```python
from build123d import *

# Parameters (mm, degrees)
CROQUIS1_W                 = 105
CROQUIS1_H                 = 30
CROQUIS1_R                 = 5
SALIENTE_EXTRUIR1_DEPTH    = 70
CORTAR_EXTRUIR1_DEPTH      = 30
CORTAR_EXTRUIR1_DEPTH_BACK = 30
CROQUIS2_R                 = 40
CROQUIS3_R                 = 5
CORTAR_EXTRUIR2_DEPTH      = 30
CROQUIS4_W                 = 55
CROQUIS4_H                 = 60
CORTAR_EXTRUIR3_DEPTH      = 30


with BuildPart() as part:
    # Croquis1 → Saliente-Extruir1 (new body)
    with BuildSketch(Plane(origin=(0, 0, 0), x_dir=(1, 0, 0), z_dir=(0, 1, 0))):
        with Locations((14.264686972, 6.108870968)):
            Rectangle(CROQUIS1_W, CROQUIS1_H)
        with Locations(Location((56.764686972, 6.108870968, 0), (0, 0, 270))):
            Circle(CROQUIS1_R, mode=Mode.SUBTRACT)
    extrude(amount=SALIENTE_EXTRUIR1_DEPTH)

    # Croquis2 → Cortar-Extruir1 (cut, two sides: drawn at the far end of the back side and taken through both)
    with BuildSketch(Plane(origin=(0, 35, 0), x_dir=(-1, 0, 0), z_dir=(0, -1, 0)).offset(-CORTAR_EXTRUIR1_DEPTH_BACK)):
        with Locations((-66.764686972, 6.108870968)):
            Circle(CROQUIS2_R)
    extrude(amount=CORTAR_EXTRUIR1_DEPTH + CORTAR_EXTRUIR1_DEPTH_BACK, mode=Mode.SUBTRACT)

    # Croquis3 → Cortar-Extruir2 (cut)
    with BuildSketch(Plane.ZY.offset(38.235313028)):
        with Locations((-6.108870968, 35)):
            Circle(CROQUIS3_R)
    extrude(amount=-CORTAR_EXTRUIR2_DEPTH, mode=Mode.SUBTRACT)

    # Croquis4 → Cortar-Extruir3 (cut)
    with BuildSketch(Plane.XY.offset(8.891129032)):
        with Locations((-5.735313028, 35)):
            Rectangle(CROQUIS4_W, CROQUIS4_H)
    extrude(amount=-CORTAR_EXTRUIR3_DEPTH, mode=Mode.SUBTRACT)


solid = part.part
```
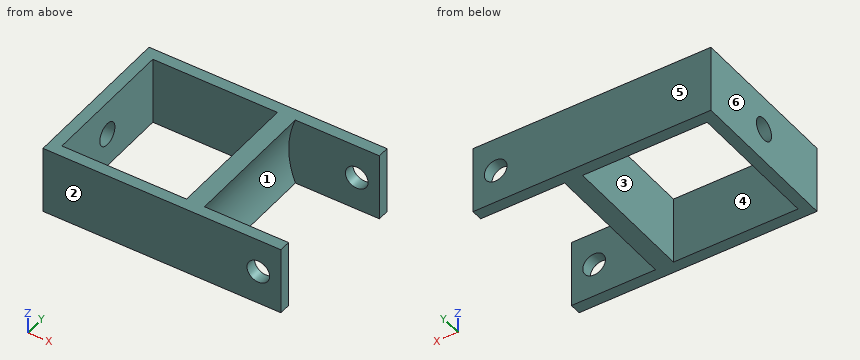
Here's how the part is built. I have some questions about the finished solid (model axes, mm). Face numbers are marked on the shaded views. A direction names the side the tool comes from. Coordinates: 2 decimals unless noted, no trailing zeros. Order: outer loops, then holes, each group sorted by start corner. A loop starts at its lowest first (then second) coordinate and runs counter-clockwise, first axis right, second up. Notation, with made-up numbers: M -22,-39 L 6,-39 A15 ccw 6,-18 Z; hole C 58,53.5 d4. An arc over 180 degrees is marked long. Answer as a JSON object with one key per item and string values. Group by question number.
(1) Suppose I cut it at B-B, the plane x = 10. Please give me the cut outline in (y, z).
(2) For pin 1 (15 mm diameter, centred on y = 34.5, z = -10, fed in from +X); pin 2 (2 mm diameter, centred on y = 9.5, z = -7.5, fed in from +X); pin 3 (6 mm diameter, centred on y = 35, z = -6.11, fed in from -X), each with a flat end and sliding along its axis, tell me the tip position at first contact or that it passes through.
(3) I need wall thicknesses on probe 1 along Y at (x, z) = (53, -17); probe 2 along Z at (x, y) = (56.5, 66.5); probe 3 along X at (y, z) = (11.5, -7). Which ranges of each line are inside material? Lowest first, please.
(4) If we mould it in two halves opening along X, with no side actions, what happens to the marked faces 4, 5 and 6? For each: released by +X, released by -X, zero draft, split by the parting line, or undercut.
(5) Which directions (+Z, -Z, +X, -X, +Y, -Y) give clear straight access to the entire face, cutting with the end or side of a thin tool? Please do the marked faces 1, 2 and 3.
(6) Suppose I cut it at A-A, the plane y = 49. Please give me the cut outline in (x, z), then the cut area to 3 significant figures.
(7) Suppose I cut it at D-D, the plane z = -17. Please give me the cut outline in (x, y), then the cut area to 3 significant figures.
(8) Suppose I cut it at C-C, the plane y = 35. Please give me the cut outline in (x, z), then the cut area to 3 significant figures.
Values found:
{
 "1": {"outline": "M 0,-21.11 L 5,-21.11 L 5,8.89 L 0,8.89 Z; M 65,-21.11 L 70,-21.11 L 70,8.89 L 65,8.89 Z"},
 "2": {"pin 1": "stops at x = 28.42", "pin 2": "stops at x = 26.84", "pin 3": "stops at x = 21.76"},
 "3": {"probe 1": "y = 0 to 5, 65 to 70", "probe 2": "z = -21.11 to -11.1, -1.12 to 8.89", "probe 3": "x = -38.24 to -33.24, 21.76 to 26.77"},
 "4": {"face 4": "undercut", "face 5": "zero draft", "face 6": "released by -X"},
 "5": {"face 1": "+X", "face 2": "+Z, -Z, +X, -X, -Y", "face 3": "+Z, -Z"},
 "6": {"outline": "M -38.24,-21.11 L -33.24,-21.11 L -33.24,8.89 L -38.24,8.89 Z; M 21.76,-21.11 L 29.68,-21.11 A40 cw 29.68,8.89 L 21.76,8.89 Z", "area": "329 mm^2"},
 "7": {"outline": "M -38.24,0 L 66.76,0 L 66.76,5 L 28.28,5 L 28.28,65 L 66.76,65 L 66.76,70 L -38.24,70 Z; hole M -33.24,5 L 21.76,5 L 21.76,65 L -33.24,65 Z", "area": "1,740 mm^2"},
 "8": {"outline": "M -38.24,-21.11 L -33.24,-21.11 L -33.24,-11.11 L -38.24,-11.11 Z; M -38.24,-1.11 L -33.24,-1.11 L -33.24,8.89 L -38.24,8.89 Z; M 21.76,-21.11 L 29.68,-21.11 A40 cw 29.68,8.89 L 21.76,8.89 Z", "area": "279 mm^2"}
}
